Geometry check sheet. Reference: the model listing, model coordinates, mm. Coordinates: 2 decimals unless noted, no trailing zeros. Loops run counter-clockwise (first coordinate to the right, second up) from the corner with the lowest first, then second, coordinate; pieces in that order, holes last. Notation, with made-up numbers: M 1.25,81.25 L 58.25,81.25 A20 ccw 58.25,97.25 Z; hole C 10.5,44.25 d2. An arc over 180 degrees is marked long. Use CSV: the item, a comma, the result in double quotes.
```python
from build123d import *

# Parameters (mm, degrees)
SKETCH1_R           = 1.575
BOSS_EXTRUDE1_DEPTH = 3.175


with BuildPart() as part:
    # Sketch1 → Boss-Extrude1 (new body)
    with BuildSketch(Plane.XY):
        Polygon((55, 75), (5, 75), (5, 71.825), (0, 71.825), (0, 50.825), (3.175, 50.825), (3.175, 29.825), (0, 29.825), (0, 8.825), (3.175, 8.825), (3.175, 0), (55, 0), (55, 8.825), (105, 8.825), (105, 0), (155, 0), (155, 8.825), (205, 8.825), (205, 0), (256.825, 0), (256.825, 8.825), (260, 8.825), (260, 29.825), (256.825, 29.825), (256.825, 50.825), (260, 50.825), (260, 71.825), (255, 71.825), (255, 75), (205, 75), (205, 71.825), (155, 71.825), (155, 75), (105, 75), (105, 71.825), (55, 71.825), align=None)
        with Locations((29.0875, 7.2375)):
            Circle(SKETCH1_R, mode=Mode.SUBTRACT)
        with Locations((230.9125, 7.2375)):
            Circle(SKETCH1_R, mode=Mode.SUBTRACT)
    extrude(amount=BOSS_EXTRUDE1_DEPTH)


solid = part.part
```
1. Section check B-B, the plane z = 1.4. Count the separate pieces of the cut face and the enclosed holes in it, plus the area to 3 significant figures.
The answers:
separate pieces,"1"
enclosed holes,"2"
area,"18,100 mm^2"
2. Section check A-A, the plane x = 201. Record the cut outline in (y, z) (3 decimals).
The answers:
outline,"M 8.825,0 L 71.825,0 L 71.825,3.175 L 8.825,3.175 Z"
3. Thickness scan on line 1 (X direction, y = 7, z = 2) (1 decimal); line 2 (X direction, y = 32.5, z = 2.6) (3 decimals); line 3 (Y direction, x = 231.5, z = 1.15). Record the ranges inside material, lowest first. Write a range as [from, to].
The answers:
line 1,"[3.2, 27.5], [30.6, 55], [105, 155], [205, 229.4], [232.5, 256.8]"
line 2,"[3.175, 256.825]"
line 3,"[0, 5.78], [8.7, 75]"
4. Gauge pin test, flat ends, axial feed: P1, Ø1, axis at y = 4, z = 2, coming from the -X side (3 decimals); P2, Ø1.6, axis at x = 190.5, z = 1, coming from the +Y side (3 decimals); P3, Ø1.5, axis at x = 175, z = 2.5, coming from the -Y side (3 decimals). Record the tip position at first contact, or that the pin passes through.
The answers:
P1,"x = 3.175"
P2,"y = 71.825"
P3,"y = 8.825"
